Input: part model. Units: mm. Frame: model coordinates. Round coordinates to 2 decimals unless told otherwise and drop trailing zeros. Loops run counter-clockwise (first coordinate to the right, second up) from the corner with the lowest first, then second, coordinate; pieces in that order, holes last. Notation, with made-up numbers: (37.25, 14.25) -> (86.25, 14.25) arc R6 cw to (86.25, 23.25) -> close; hole circle Ø3 at (33.5, -13.5). An arc over 180 degrees is marked (long way). One line per question, with ' | ' between items. Start each with the question number.
Q1. Contact query for flat-ended pins moving along their axis: P1, Ø1.5, axis at x = -55, z = 0.5, coming from the +Y side; P2, Ø1.5, axis at y = 35, z = 1, coming from the -X side; P3, Ø11, axis at x = 29.78, y = 70.43, coming from the +Z side. Output: stop coordinate, or through.
Q2. Cut plane A-A on x = -32.5. Return loops of the section in (y, z) (3 decimals), and give its area (3 significant figures).
Q3. Cut plane C-C on y = 86. Return loops of the section in (x, z) (3 decimals).
Q4. Material intervals for L1, parallel to X at y = 50.5, z = 1.6; L2, parallel to X at y = 21, z = 1.7; L3, parallel to X at y = 74.5, z = 1.85, sorted ascending.
Q5. Cut plane B-B on z = 1.25. Return loops of the section in (x, y).
from build123d import *

# Parameters (mm, degrees)
F1_DEPTH = 3.175


with BuildPart() as f1:
    # F0 (on Top) → F1 (new body)
    with BuildSketch(Plane.XY):
        with BuildLine():
            Line((0, 82.8428900972), (0, 101.6198892983))
            ThreePointArc((0, 101.6198892983), (-71.8561128263, 71.8561128263), (-101.6198892983, 0))
            Line((-101.6198892983, 0), (-83.0405046204, 0))
            ThreePointArc((-83.0405046204, 0), (-81.0138961368, 4.747652407), (-76.1835112753, 6.5682916938))
            ThreePointArc((-76.1835112753, 6.5682916938), (-75.3538778245, 12.9947275008), (-73.9831338439, 19.3278491468))
            ThreePointArc((-73.9831338439, 19.3278491468), (-78.1170647151, 27.5165370514), (-69.7636527981, 31.306590269))
            ThreePointArc((-69.7636527981, 31.306590269), (-65.9297039839, 38.7342739522), (-61.3079271878, 45.6991018505))
            ThreePointArc((-61.3079271878, 45.6991018505), (-62.070439488, 55.1904658501), (-52.5550284868, 55.5431258281))
            ThreePointArc((-52.5550284868, 55.5431258281), (-44.6644810596, 62.0657230497), (-35.973351178, 67.4758316068))
            ThreePointArc((-35.973351178, 67.4758316068), (-32.4523110588, 76.7481303158), (-23.3473151394, 72.8146463412))
            ThreePointArc((-23.3473151394, 72.8146463412), (-14.9553750219, 74.9893766074), (-6.3712090649, 76.200246332))
            ThreePointArc((-6.3712090649, 76.200246332), (-4.6020924898, 80.8801750033), (0, 82.8428900972))
        make_face()
        with BuildLine():
            Line((83.0405046204, 0), (101.6198892983, 0))
            ThreePointArc((101.6198892983, 0), (71.8561128263, 71.8561128263), (0, 101.6198892983))
            Line((0, 101.6198892983), (0, 82.8428900972))
            ThreePointArc((0, 82.8428900972), (4.509046567, 80.9751818558), (6.3767548084, 76.4661352888))
            ThreePointArc((6.3767548084, 76.4661352888), (6.3753682218, 76.3331618962), (6.3712090649, 76.200246332))
            ThreePointArc((6.3712090649, 76.200246332), (14.9553750219, 74.9893766074), (23.3473151394, 72.8146463412))
            ThreePointArc((23.3473151394, 72.8146463412), (30.9922218938, 77.1819499048), (36.641312364, 70.4287494368))
            ThreePointArc((36.641312364, 70.4287494368), (36.4722388851, 68.9149879086), (35.973351178, 67.4758316068))
            ThreePointArc((35.973351178, 67.4758316068), (44.6644810596, 62.0657230497), (52.5550284868, 55.5431258281))
            ThreePointArc((52.5550284868, 55.5431258281), (59.71374592, 56.8808501906), (63.7362883578, 50.8099446492))
            ThreePointArc((63.7362883578, 50.8099446492), (63.0983300746, 47.9807375127), (61.3079271878, 45.6991018505))
            ThreePointArc((61.3079271878, 45.6991018505), (65.9297039839, 38.7342739522), (69.7636527981, 31.306590269))
            ThreePointArc((69.7636527981, 31.306590269), (75.6863195554, 30.6673507833), (78.478089889, 25.4049723246))
            ThreePointArc((78.478089889, 25.4049723246), (77.232242702, 21.625552529), (73.9831338439, 19.3278491468))
            ThreePointArc((73.9831338439, 19.3278491468), (75.3538778245, 12.9947275008), (76.1835112753, 6.5682916938))
            ThreePointArc((76.1835112753, 6.5682916938), (81.0138961368, 4.747652407), (83.0405046204, 0))
        make_face()
        with BuildLine():
            ThreePointArc((6.3712090649, 76.200246332), (4.4140397145, 71.864042799), (0, 70.0893804804))
            Line((0, 70.0893804804), (0, 0))
            Line((0, 0), (27.1081153594, 64.1093685577))
            ThreePointArc((27.1081153594, 64.1093685577), (23.4817449036, 67.7077241487), (23.3473151394, 72.8146463412))
            ThreePointArc((23.3473151394, 72.8146463412), (14.9553750219, 74.9893766074), (6.3712090649, 76.200246332))
        make_face()
        with BuildLine():
            ThreePointArc((0, 70.0893804804), (-4.4140397145, 71.864042799), (-6.3712090649, 76.200246332))
            ThreePointArc((-6.3712090649, 76.200246332), (-14.9553750219, 74.9893766074), (-23.3473151394, 72.8146463412))
            ThreePointArc((-23.3473151394, 72.8146463412), (-23.0270127411, 71.6407581215), (-22.9191140542, 70.4287494368))
            ThreePointArc((-22.9191140542, 70.4287494368), (-24.0614629124, 66.6378950928), (-27.1081153594, 64.1093685577))
            Line((-27.1081153594, 64.1093685577), (0, 0))
            Line((0, 0), (0, 70.0893804804))
        make_face()
        with BuildLine():
            Line((52.217256626, 46.4294234482), (0, 0))
            Line((0, 0), (66.1279660789, 23.2934075977))
            ThreePointArc((66.1279660789, 23.2934075977), (66.3348002352, 28.0309350677), (69.7636527981, 31.306590269))
            ThreePointArc((69.7636527981, 31.306590269), (65.9297039839, 38.7342739522), (61.3079271878, 45.6991018505))
            ThreePointArc((61.3079271878, 45.6991018505), (56.6159288766, 44.2386760913), (52.217256626, 46.4294234482))
        make_face()
        with BuildLine():
            ThreePointArc((69.8917659573, 0), (71.7184828819, 4.547760848), (76.1835112753, 6.5682916938))
            ThreePointArc((76.1835112753, 6.5682916938), (75.3538778245, 12.9947275008), (73.9831338439, 19.3278491468))
            ThreePointArc((73.9831338439, 19.3278491468), (69.2582948104, 19.7313872539), (66.1279660789, 23.2934075977))
            Line((66.1279660789, 23.2934075977), (0, 0))
            Line((0, 0), (69.8917659573, 0))
        make_face()
        with BuildLine():
            Line((-52.217256626, 46.4294234482), (0, 0))
            Line((0, 0), (-27.1081153594, 64.1093685577))
            ThreePointArc((-27.1081153594, 64.1093685577), (-32.215926502, 64.014547821), (-35.973351178, 67.4758316068))
            ThreePointArc((-35.973351178, 67.4758316068), (-44.6644810596, 62.0657230497), (-52.5550284868, 55.5431258281))
            ThreePointArc((-52.5550284868, 55.5431258281), (-51.0729425155, 53.3798425122), (-50.5514077561, 50.8099446492))
            ThreePointArc((-50.5514077561, 50.8099446492), (-50.9819275359, 48.4666553772), (-52.217256626, 46.4294234482))
        make_face()
        with BuildLine():
            Line((-66.1279660789, 23.2934075977), (0, 0))
            Line((0, 0), (-52.217256626, 46.4294234482))
            ThreePointArc((-52.217256626, 46.4294234482), (-56.6159288766, 44.2386760913), (-61.3079271878, 45.6991018505))
            ThreePointArc((-61.3079271878, 45.6991018505), (-65.9297039839, 38.7342739522), (-69.7636527981, 31.306590269))
            ThreePointArc((-69.7636527981, 31.306590269), (-66.8601369383, 28.968776483), (-65.7669409051, 25.4049723246))
            ThreePointArc((-65.7669409051, 25.4049723246), (-65.8578473348, 24.3338695317), (-66.1279660789, 23.2934075977))
        make_face()
        with BuildLine():
            ThreePointArc((-73.9831338439, 19.3278491468), (-75.3538778245, 12.9947275008), (-76.1835112753, 6.5682916938))
            ThreePointArc((-76.1835112753, 6.5682916938), (-71.7184828819, 4.547760848), (-69.8917659573, 0))
            Line((-69.8917659573, 0), (0, 0))
            Line((0, 0), (-66.1279660789, 23.2934075977))
            ThreePointArc((-66.1279660789, 23.2934075977), (-69.2582948104, 19.7313872539), (-73.9831338439, 19.3278491468))
        make_face()
        with BuildLine():
            Line((27.1081153594, 64.1093685577), (0, 0))
            Line((0, 0), (52.217256626, 46.4294234482))
            ThreePointArc((52.217256626, 46.4294234482), (50.5559307535, 51.0541059125), (52.5550284868, 55.5431258281))
            ThreePointArc((52.5550284868, 55.5431258281), (44.6644810596, 62.0657230497), (35.973351178, 67.4758316068))
            ThreePointArc((35.973351178, 67.4758316068), (32.215926502, 64.014547821), (27.1081153594, 64.1093685577))
        make_face()
    extrude(amount=F1_DEPTH)


solid = f1.part
Results:
1) P1: y = 85.93 | P2: x = -95.67 | P3: through
2) outline: (0, 0) -> (64.13, 0) -> (64.13, 3.175) -> (0, 3.175) -> close; (76.728, 0) -> (96.283, 0) -> (96.283, 3.175) -> (76.728, 3.175) -> close | area: 266 mm^2
3) outline: (-54.135, 0) -> (54.135, 0) -> (54.135, 3.175) -> (-54.135, 3.175) -> close
4) L1: -88.18 to -63.73, -50.56 to 50.56, 63.73 to 88.18 | L2: -99.43 to -76.7, -67.54 to 67.54, 76.7 to 99.43 | L3: -69.11 to -35.3, -24.26 to -6.07, 6.07 to 24.26, 35.3 to 69.11
5) outline: (-101.62, 0) -> (-83.04, 0) arc R6.57 cw to (-69.89, 0) -> (69.89, 0) arc R6.57 cw to (83.04, 0) -> (101.62, 0) arc R101.62 ccw to start; hole circle Ø12.71 at (-72.12, 25.4); hole circle Ø13.18 at (-57.14, 50.81); hole circle Ø13.72 at (-29.78, 70.43); hole circle Ø12.75 at (0, 76.47); hole circle Ø13.72 at (29.78, 70.43); hole circle Ø13.18 at (57.14, 50.81); hole circle Ø12.71 at (72.12, 25.4)
